```python
from build123d import *

# Parameters (mm, degrees)
CROQUIS1_R              = 9.906
SALIENTE_EXTRUIR1_DEPTH = 367.538
CROQUIS2_R              = 3.1
CORTAR_EXTRUIR1_DEPTH   = 10
CROQUIS3_R              = 10.5
SALIENTE_EXTRUIR2_DEPTH = 2


with BuildPart() as part:
    # Croquis1 → Saliente-Extruir1 (new body)
    with BuildSketch(Plane(origin=(0, 0, 0), x_dir=(1, 0, 0), z_dir=(0, 1, 0))):
        Circle(CROQUIS1_R)
    extrude(amount=SALIENTE_EXTRUIR1_DEPTH)

    # Croquis2 → Cortar-Extruir1 (cut, symmetric)
    with BuildSketch(Plane.XY):
        with Locations((0, 358.648)):
            Circle(CROQUIS2_R)
    extrude(amount=CORTAR_EXTRUIR1_DEPTH, both=True, mode=Mode.SUBTRACT)

    # Croquis3 → Saliente-Extruir2 (add)
    with BuildSketch(Plane.XZ):
        Circle(CROQUIS3_R)
    extrude(amount=SALIENTE_EXTRUIR2_DEPTH)


solid = part.part
```
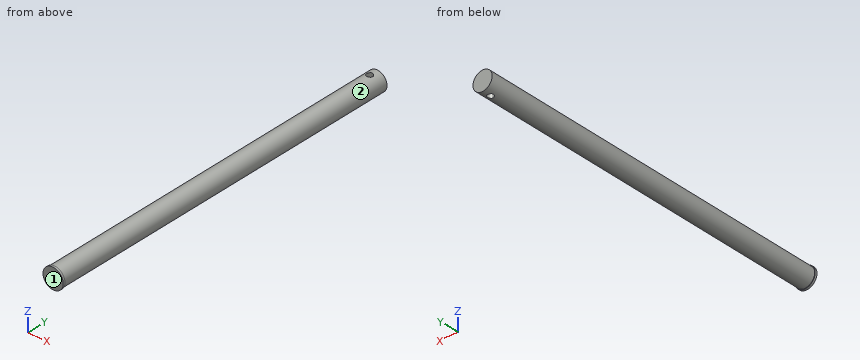
Input: part model. Units: mm. Frame: model coordinates. Face numbers are marked on the shaded views. A direction names the side the tool comes from. Coordinates: 2 decimals unless noted, no trailing zeros. Write each loop counter-clockwise with the first axis right and the second up, starting at its lowest first coordinate (ties: lowest second). Pieces come first, ordered by that corner, then holes.
1) Pin query (flat end, axial travel): pin 1 Ø10 at (x, y) = (0, 358.648) entering from +Z; pin 2 Ø3 at (x, y) = (4.5, 234) entering from -Z; pin 3 Ø8 at (y, z) = (41.5, -1) entering from -X. Return the tip coordinate at first contact, or that it passes through.
2) Material intervals for line 1 along Y through (x, z) = (0, 3.75); line 2 along Y through (x, z) = (0.25, 0.75); line 3 along Y through (x, z) = (-6, -8), sorted ascending.
3) Set-up query: the marked faces 1 and 2. Return all of +Z, -Z, +X, -X, +Y, -Y with unobstructed straight access to the full face (end or side cutting, diameter ignored); none if empty.
4) Section B-B on z = -3.75. Output: boundary loops of the cut face in (x, y), and give its area (3 significant figures).
5) Section A-A on x = 0. Output: boundary loops of the cut face in (y, z), and give its area (3 significant figures).
6) Section C-C on y = 206. Output: boundary loops of the cut face in (x, z), and give its area (3 significant figures).
Check result:
1. pin 1: stops at z = 9.91
1. pin 2: stops at z = -9.44
1. pin 3: stops at x = -9.91
2. line 1: y = -2 to 355.55, 361.75 to 367.54
2. line 2: y = -2 to 355.56, 361.74 to 367.54
2. line 3: y = -2 to 0
3. face 1: +Z, -Z, +X, -X, -Y
3. face 2: +Y
4. outline: (-9.81, -2) - (9.81, -2) - (9.81, 0) - (9.17, 0) - (9.17, 367.54) - (-9.17, 367.54) - (-9.17, 0) - (-9.81, 0) - close; hole circle Ø6.2 at (0, 358.65)
4. area: 6,750 mm2
5. outline: (-2, -10.5) - (0, -10.5) - (0, -9.91) - (355.55, -9.91) - (355.55, 9.91) - (0, 9.91) - (0, 10.5) - (-2, 10.5) - close; (361.75, -9.91) - (367.54, -9.91) - (367.54, 9.91) - (361.75, 9.91) - close
5. area: 7,200 mm2
6. outline: circle Ø19.81 at (0, 0)
6. area: 308 mm2
